Part model, mm, in its own coordinate system. Face numbers are marked on the shaded views. A direction names the side the tool comes from. Coordinates: 2 decimals unless noted, no trailing zeros. Loops run counter-clockwise (first coordinate to the right, second up) from the corner with the lowest first, then second, coordinate; pieces in that order, holes last. Notation, with made-up numbers: (50, -28) - (68, -28) arc R16 ccw to (68, -3) - close; hole circle Ø1 at (-34, 72.25). An arc over 180 degrees is marked (long way). Use a Markdown table: item, result. Add a question column.
1. Band-saw the part on A-A, the plane y = -3.5. Give the cut face in (x, z), plus the area to 3 significant figures.
2. Drop flat-ended pins along their axis: pin 1 (1 mm diameter, centred on y = -3.5, z = 1, fed in from +X); pin 2 (3.5 mm diameter, centred on x = -1.5, z = -0.5, fed in from +Y); pin 3 (1.5 mm diameter, centred on y = 2.5, z = 2, fed in from -X); pin 4 (2 mm diameter, centred on y = -6.5, z = 1.5, fed in from -X). Give the stop position or say it passes through.
3. Band-saw the part on D-D, the plane x = -3. Give the cut face in (y, z).
4. 3-axis set-ups, long thin cutter, end or side, ignore diameter. For the marked faces 1 and 2: which of +Z, -Z, +X, -X, +Y, -Y reach the whole face in a straight line?
5. Band-saw the part on C-C, the plane y = 1.5. Give the cut face in (x, z).
6. Band-saw the part on B-B, the plane x = 0. Count the separate pieces of the cut face and the enclosed holes in it, plus the area to 3 significant figures.
7. Pull direction Z, two halves, no side cores. Call the marked faces 3, 4 and 5: pulls with the +Z half, pulls with the -Z half, needs draft (parallel to the pull), parting line crosses it, or undercut.
8. Wall check: probe 1 along Y at (x, z) = (0.55, 0); probe 2 along Y at (x, z) = (-0.5, 0); probe 3 along Y at (x, z) = (-0.5, 3). Give the ranges that are in metal, low to high. Write a range as [from, to].
from build123d import *

# Parameters (mm, degrees)
SKETCH1_R                 = 1
BOSS_EXTRUDE1_DEPTH       = 5
SKETCH2_R                 = 3.5
BOSS_EXTRUDE2_DEPTH       = 9
F_3_0MM_DOWEL_HOLE1_D     = 3.1
F_3_0MM_DOWEL_HOLE2_D     = 2.5
F_3_0MM_DOWEL_HOLE2_DEPTH = 3
F_3_0MM_DOWEL_HOLE2_TIP   = 0.751075774
F_1_0MM_DOWEL_HOLE1_D     = 1
FILLET1_R                 = 1


with BuildPart() as part:
    # Sketch1 → Boss-Extrude1 (new body)
    with BuildSketch(Plane(origin=(0, 0, 0), x_dir=(1, 0, 0), z_dir=(0, 1, 0))):
        with Locations(Location((0, 0, 0), (0, 0, 270))):
            Circle(SKETCH1_R)
    extrude(amount=BOSS_EXTRUDE1_DEPTH)

    # Sketch2 → Boss-Extrude2 (add)
    with BuildSketch(Plane.XZ):
        with Locations(Location((0, 0, 0), (0, 0, 270))):
            Circle(SKETCH2_R)
    extrude(amount=BOSS_EXTRUDE2_DEPTH)

    # Ø3.0mm Dowel Hole1 (through all)
    with Locations(Plane(origin=(0.004438696, -4.500949112, 3.499997185), x_dir=(0.999999195836, 0, -0.001268198744), z_dir=(0.001268198744, 0, 0.999999195836))):
        with Locations((0, 0)):
            Hole(F_3_0MM_DOWEL_HOLE1_D / 2)

    # Ø3.0mm Dowel Hole2
    with Locations(Plane(origin=(3.499992934, -4.513990385, 0.007032841), x_dir=(-0.002009383102, 0, 0.999997981188), z_dir=(0.999997981188, 0, 0.002009383102))):
        with Locations((0, 0)):
            Hole(F_3_0MM_DOWEL_HOLE2_D / 2, depth=F_3_0MM_DOWEL_HOLE2_DEPTH)
            with Locations((0, 0, -(F_3_0MM_DOWEL_HOLE2_DEPTH + F_3_0MM_DOWEL_HOLE2_TIP / 2))):  # 118° drill point
                Cone(0, F_3_0MM_DOWEL_HOLE2_D / 2, F_3_0MM_DOWEL_HOLE2_TIP, mode=Mode.SUBTRACT)

    # Ø1.0mm Dowel Hole1 (through all)
    with Locations(Plane(origin=(1, 3.476098955, 0), x_dir=(0, 0, 1), z_dir=(1, 0, 0))):
        with Locations((0, 0)):
            Hole(F_1_0MM_DOWEL_HOLE1_D / 2)

    # Fillet1
    fillet1_edges = [part.edges().sort_by_distance(p)[0] for p in [
        (0, 0, -1),
    ]]
    fillet(fillet1_edges, radius=FILLET1_R)


solid = part.part
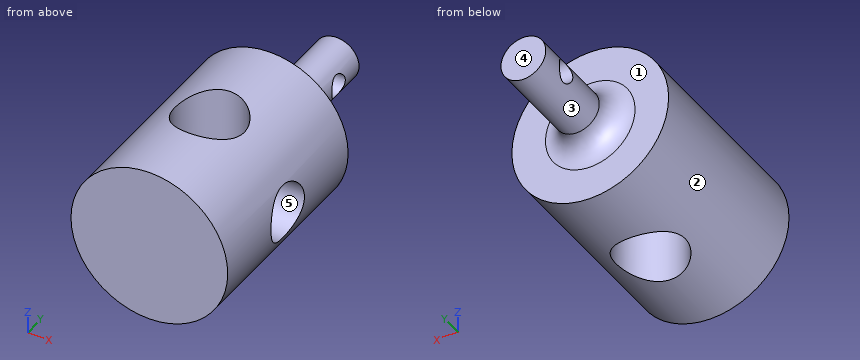
Geometry check:
| question | item | result |
|---|---|---|
| 1 | outline | (-1.19, -3.29) - (-1.18, 3.3) arc R3.5 ccw to start; (1.18, -3.3) arc R3.5 ccw to (3.42, -0.72) - (1.18, -0.73) - close; (1.18, 0.73) - (3.42, 0.74) arc R3.5 ccw to (1.19, 3.29) - close |
| 1 | area | 18.9 mm^2 |
| 2 | pin 1 | stops at x = 3.46 |
| 2 | pin 2 | stops at y = 5 |
| 2 | pin 3 | passes through |
| 2 | pin 4 | stops at x = -3.46 |
| 3 | outline | (-9, -1.8) - (0, -1.8) - (0, 1.8) - (-9, 1.8) - close |
| 4 | face 1 | +Y |
| 4 | face 2 | +Y, -Y |
| 5 | outline | circle Ø2 at (0, 0) |
| 6 | separate pieces | 2 |
| 6 | enclosed holes | 1 |
| 6 | area | 50.9 mm^2 |
| 7 | face 3 | parting line crosses it |
| 7 | face 4 | needs draft |
| 7 | face 5 | undercut |
| 8 | probe 1 | y = [-9, -5.95], [-3.05, 2.98], [3.98, 5] |
| 8 | probe 2 | y = [-9, -5.97], [-3.03, 2.98], [3.98, 5] |
| 8 | probe 3 | y = [-9, -5.97], [-3.04, 0] |
